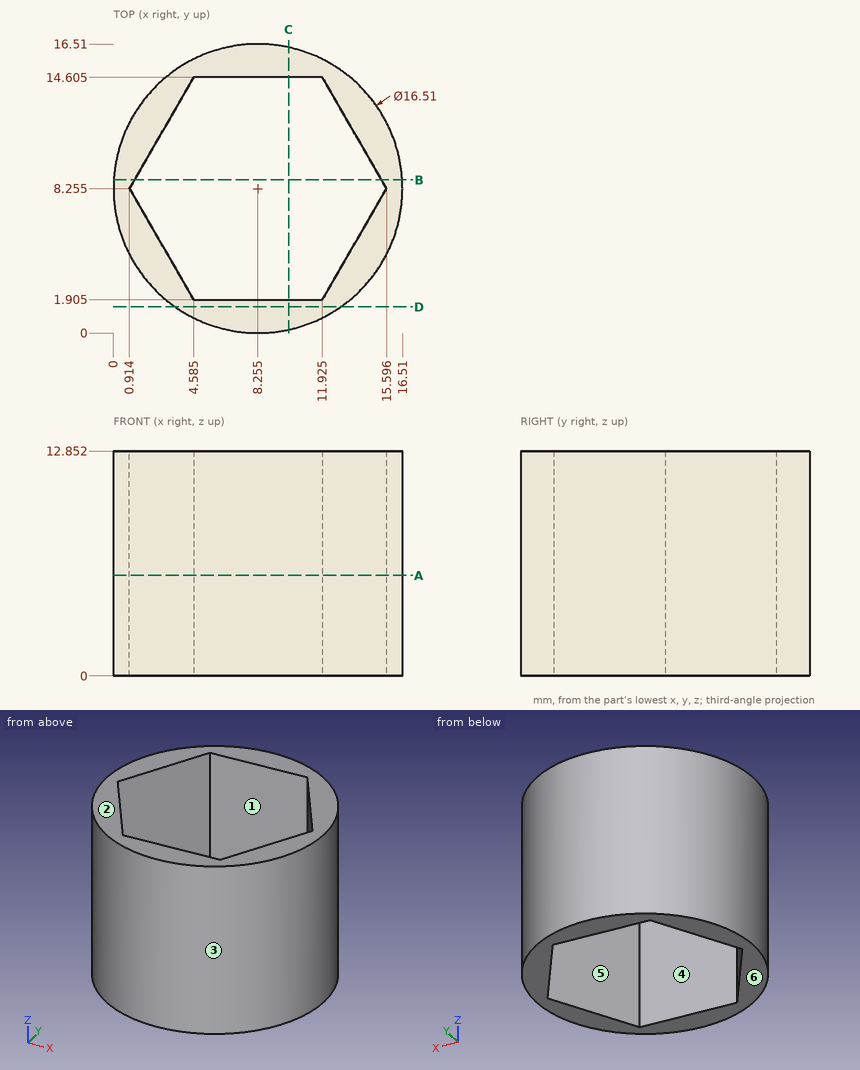
Verification items for this drawing (mm, ordinates from the low corner). A direction names the side the tool comes from. Round coordinates to 2 decimals unless told otherwise and drop trailing zeros. Order: outer loops, then holes, each group sorted by start corner. A loop starts at its lowest first (then second) coordinate and runs counter-clockwise, first axis right, second up. Notation, with made-up numbers: M 16.25,7 L 34.25,7 A20 ccw 34.25,19 Z; hole C 74.25,-21 d5. An arc over 180 degrees is marked long. Answer in a Markdown table with one row per item. Add a question column.
Item 1: Sectioned sample at D-D, the plane y = 1.5. Enter the section's corners in (x, z), plus the area to 3 significant figures.
Item 2: Sectioned sample at C-C, the plane x = 10. Enter the section's corners in (y, z) (1 decimal).
Item 3: Depth check by flat-ended pin: pin 1 Ø3 at (y, z) = (12.5, 7) entering from +X; pin 2 Ø2 at (x, z) = (9.5, 4) entering from +Y; pin 3 Ø1.5 at (y, z) = (12.5, 8.5) entering from -X. Enter the tip coordinate at first touch or a pass-through.
Item 4: Material ranges on L1, parallel to Y at x = 8.25, z = 5.75 (1 decimal); L2, parallel to X at y = 8, z = 1.5 (1 decimal); L3, parallel to X at y = 2, z = 9.5, recorded low to high. Write a range as [from, to].
Item 5: Set-up check for the marked faces 5 and 6: record each of +Z, -Z, +X, -X, +Y, -Y from which the full face is reachable in a straight line by a thin tool's end or side.
Item 6: Draft check along X on the marked faces 1, 2, 3 and 4. Enter one of: released by +X, released by -X, zero draft, split by the parting line, or undercut.
Item 7: Sectioned sample at A-A, the plane z = 5.75. Enter the section's corners in (x, y) (1 decimal).
Item 8: Sectioned sample at B-B, the plane y = 8.75. Enter the section's corners in (x, z) (1 decimal).
Filled in:
| question | item | result |
|---|---|---|
| 1 | outline | M 3.51,0 L 13,0 L 13,12.85 L 3.51,12.85 Z |
| 1 | area | 122 mm² |
| 2 | outline | M 0.2,0 L 1.9,0 L 1.9,12.9 L 0.2,12.9 Z; M 14.6,0 L 16.3,0 L 16.3,12.9 L 14.6,12.9 Z |
| 3 | pin 1 | stops at x = 16.04 |
| 3 | pin 2 | stops at y = 16.51 |
| 3 | pin 3 | stops at x = 0.78 |
| 4 | L1 | y = [0, 1.9], [14.6, 16.5] |
| 4 | L2 | x = [0, 1.1], [15.4, 16.5] |
| 4 | L3 | x = [2.87, 4.53], [11.98, 13.64] |
| 5 | face 5 | +Z, -Z |
| 5 | face 6 | -Z, +X, -X, +Y, -Y |
| 6 | face 1 | undercut |
| 6 | face 2 | zero draft |
| 6 | face 3 | split by the parting line |
| 6 | face 4 | undercut |
| 7 | outline | C 8.3,8.3 d16.5; hole M 0.9,8.3 L 4.6,1.9 L 11.9,1.9 L 15.6,8.3 L 11.9,14.6 L 4.6,14.6 Z |
| 8 | outline | M 0,0 L 1.2,0 L 1.2,12.9 L 0,12.9 Z; M 15.3,0 L 16.5,0 L 16.5,12.9 L 15.3,12.9 Z |
